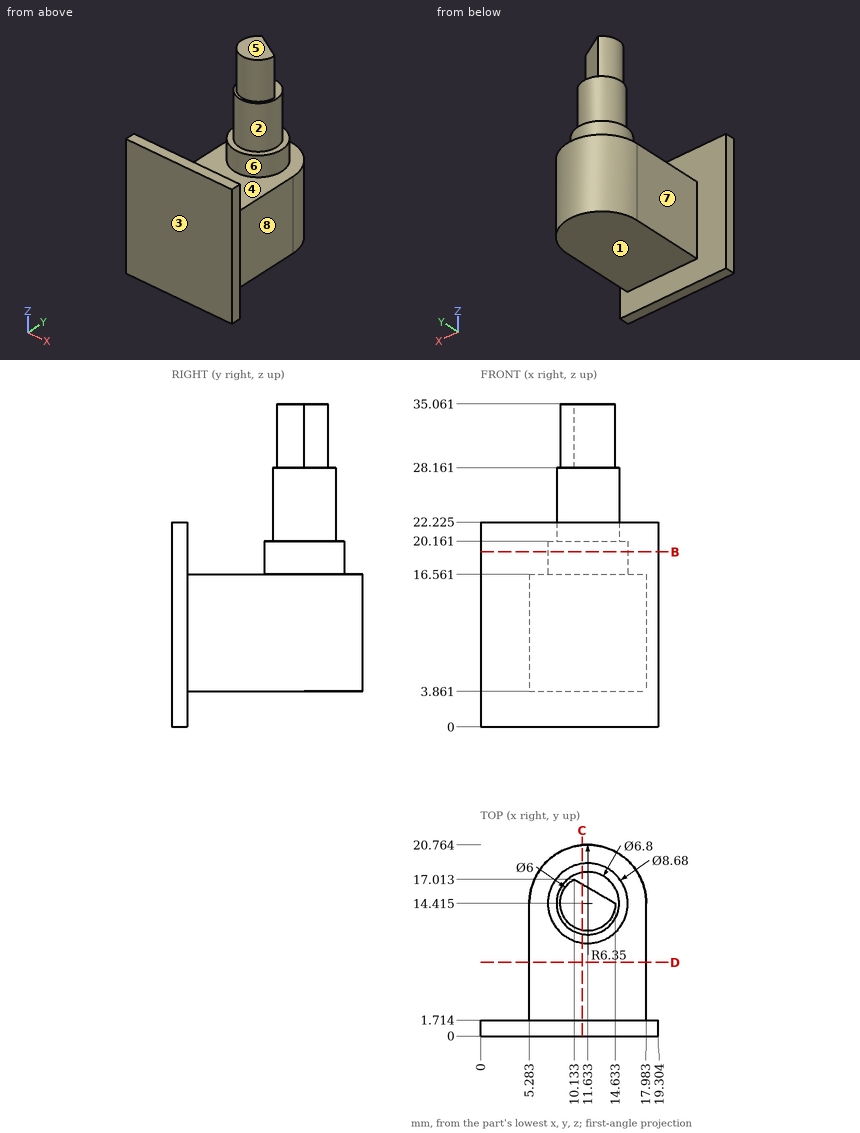
Design review of the part shown in the three views and the two pictorial views. Dimensions are in mm from the part's minimum x, y and z. A direction names the side the tool comes from. Give positions to 0.01 mm unless a question says otherwise; leave off trailing zeros. Write each loop counter-clockwise with the first axis right and the second up, starting at its lowest first coordinate (ties: lowest second). Pieces come first, ordered by that corner, then holes.
(1) Add section B-B (z = 19). Give the boundary of the cut face in (x, y) (1 decimal).
Checked values:
outline: (0, 0) - (19.3, 0) - (19.3, 1.7) - (0, 1.7) - close; circle Ø8.7 at (11.6, 14.4)
(2) Mouldability with a two-part tool opening along Y and no side actions: class the marked faces 1, 2, 3 and 4 as +Y half, -Y half, draft (parallel to the pull), parting line (faces both ways), or undercut.
Checked values:
face 1: draft
face 2: undercut
face 3: -Y half
face 4: undercut
(3) Add section D-D (y = 8). Give the boundary of the cut face in (x, z), and give its area (3 significant figures).
Checked values:
outline: (5.28, 3.86) - (17.98, 3.86) - (17.98, 16.56) - (5.28, 16.56) - close
area: 161 mm2
(4) Wall thickness on line 1 along Y through (x, z) = (11.75, 26.5); line 2 along Z through (x, y) = (7.75, 1) (1 decimal); line 3 along X through (y, z) = (11, 15.5): over which ranges is each line inside the solid? List them lowest first.
Checked values:
line 1: y = 11.02 to 17.81
line 2: z = 0 to 22.2
line 3: x = 5.28 to 17.98
(5) Clearance check with flat-ended pins moving along their axes: pin 1 Ø10 at (x, y) = (10.5, 17) entering from +Z; pin 2 Ø10 at (x, y) = (11.5, 15.5) entering from -Z; pin 3 Ø1.5 at (y, z) = (18.5, 16) entering from -X; pin 4 Ø4 at (y, z) = (11, 10) entering from +X. State where each tip first meets the part, or that it passes through.
Checked values:
pin 1: stops at z = 35.06
pin 2: stops at z = 3.86
pin 3: stops at x = 6.23
pin 4: stops at x = 17.98
(6) Tool access review of the marked faces 5, 6, 7 and 8: name each direction out of +Z, -Z, +X, -X, +Y, -Y from which nothing blocks a thin tool from reaching the whole face with its end or side.
Checked values:
face 5: +Z, +X, -X, +Y, -Y
face 6: +Z
face 7: +Z, -Z, -X, +Y
face 8: +Z, -Z, +X, +Y
(7) Add section C-C (x = 11). Give the boundary of the cut face in (y, z) (1 decimal).
Checked values:
outline: (0, 0) - (1.7, 0) - (1.7, 3.9) - (20.7, 3.9) - (20.7, 16.6) - (18.7, 16.6) - (18.7, 20.2) - (17.8, 20.2) - (17.8, 28.2) - (16.5, 28.2) - (16.5, 35.1) - (11.5, 35.1) - (11.5, 28.2) - (11.1, 28.2) - (11.1, 20.2) - (10.1, 20.2) - (10.1, 16.6) - (1.7, 16.6) - (1.7, 22.2) - (0, 22.2) - close
